Input: part model. Units: mm. Frame: model coordinates. A direction names the side the tool comes from. Give positions to 0.01 mm unless a question says otherwise; leave off trailing zeros. Loops run counter-clockwise (first coordinate to the right, second up) from the corner with the lowest first, then second, coordinate; pieces in that order, holes last. Notation, with made-up numbers: (68.25, -23.5) -> (101.25, -23.5) arc R21 cw to (101.25, 11.5) -> close; hole circle Ø8 at (43, -26.5). An arc over 180 degrees is marked (long way). Answer as a JSON object with one key per item and string values.
Autodesk Inventor part; units mm, degrees
ref_plane "Work Plane1" through (30.1625, 0, 0) normal (0, 0, -1) x (1, 0, 0)
ref_plane "YZ Plane" through (0, 0, 0) normal (1, 0, 0) x (0, 1, 0)
ref_plane "XZ Plane" through (0, 0, 0) normal (0, 1, 0) x (-1, 0, 0)
sketch "Sketch1" plane through (0, 0, 0) normal (0, 0, 1) x (1, 0, 0)
  line L0 (-7.1374, 0) -> (63.5, 0)
  line L1 (63.5, 0) -> (63.5, 6.35)
  line L2 (63.5, 6.35) -> (9.525, 6.35)
  line L3 (9.525, 6.35) -> (8.5483, 6.35)
  line L4 (8.5483, 6.35) -> (0, 6.35)
  line L5 (0, 6.35) -> (0, 12.5349)
  line L6 (-21.2649, 0) -> (77.6275, 0)
  line L7 (0, -2.507) -> (0, 15.0419)
  line L8 (-7.1374, 0) -> (-7.1374, 12.5349)
  line L9 (0, 12.5349) -> (-7.1374, 12.5349)
  line L10 (9.525, 6.35) -> (0, 6.35) construction
  dimension "d0" = 63.5
  dimension "d1" = 53.975
  dimension "d2" = 0.9767
  dimension "d3" = 7.1374
  dimension "d4" = 12.7
  dimension "d5" = 12.7
  dimension "d9" = 25.0698
  dimension "d10" = 0
revolve "Body" add sketch "Sketch1" angle 360 about axis through (-7.1374, 0, 0) along (1, 0, 0)
sketch "Sketch2" plane through (-7.1374, 0, 0) normal (-1, 0, 0) x (0, 0, 1)
  circle A0 centre (0, 0) radius 12.5349
  line L0 (0, 0) -> (0, 12.5349)
  line L1 (-12.5349, 1.3462) -> (12.5349, 1.3462)
  line L2 (12.5349, 1.3462) -> (12.5349, -1.3462)
  line L3 (12.5349, -1.3462) -> (-12.5349, -1.3462)
  line L4 (-12.5349, -1.3462) -> (-12.5349, 1.3462)
  line L5 (-12.5349, 0) -> (12.5349, 0) construction
  line L6 (0, 1.3462) -> (0, -1.3462) construction
  dimension "d11" = 2.6924
  dimension "d12" = 25.0698
fillet "Fillet1" radius 4.445 1 edges at (-7.1374, -12.5349, 0)
extrude "Slot" cut sketch "Sketch2" against normal blind 4.0894 contours A0 L3 L1 | L2 L3 A0 | A0 L1 L2 | L3 L4 A0 | A0 L4 L1
thread "Thread"
chamfer "Chamfer1" distance 0.9766 distance2 0.9767 1 edges at (63.5, -6.35, 0) measured on face at (63.5, 0.6891, 1.4726)
ref_plane "Work Plane1" through (30.1625, 0, 0) normal (0, 0, -1) x (1, 0, 0)
equation "\"d11\" = SBR"
equation "\"d12\" = KOD"
equation "\"d14\" = RR"
equation "\"d19\" = STI"
equation "\"d15\" = GEL"
equation "\"d17\" = -0.5 * SPD + 0.5 * GD"
equation "\"d0\" = NLG"
equation "\"d1\" = GEL"
equation "\"d3\" = KOH"
equation "\"d4\" = GD"
equation "\"d5\" = BDM"
equation "\"d9\" = KOD"
equation "\"GD\" = NND"
equation "\"NLG\" = 63.5"
equation "\"GEL\" = 53.975"
equation "\"KOD\" = 25.0698"
equation "\"KOH\" = 7.1374"
equation "\"GAL\" = 0.97663"
equation "\"SPD\" = GD1"
equation "\"BDM\" = NND"
equation "\"GUL\" = 0.97663"
equation "\"RR\" = 4.445"
equation "\"SBR\" = 2.6924"
equation "\"STI\" = 4.0894"
equation "\"KEWI\" = 0"
equation "\"THREADDIA\" = 12.7"
equation "\"TOA\" = 30deg"
equation "\"NND\" = 12.7"
equation "\"GD1\" = 10.74674"
properties part number "ANSI B18.6.3 - 1/2 - 13 x 2 1/2 SP HMS" material "Steel, Mild"
Q1. Access query for faces 4 (the flat face through (-3.048, 0, 0)), 5 (the flat face through (0, -6, 3)), 6 (the flat face through (-7.137, 4, 0)). Directions: +Z, -Z, +X, -X, +Y, -Y. A direction counts if a zero-diameter tool reaches every point of the face in a straight line with its end or side. Return the directions, or none.
Evaluation:
{"face 4": "+Z, -Z, -X", "face 5": "+X", "face 6": "+Z, -Z, -X, +Y, -Y"}
Q2. Section B-B, the plane z = 0. Return the cut outline in (x, y) (3 decimals).
Evaluation:
{"outline": "(-7.137, -8.09) arc R4.445 ccw to (-2.692, -12.535) -> (0, -12.535) -> (0, -6.35) -> (62.523, -6.35) -> (63.5, -5.373) -> (63.5, 5.373) -> (62.523, 6.35) -> (0, 6.35) -> (0, 12.535) -> (-2.692, 12.535) arc R4.445 ccw to (-7.137, 8.09) -> (-7.137, 1.346) -> (-3.048, 1.346) -> (-3.048, -1.346) -> (-7.137, -1.346) -> close"}
Q3. Draft query along Y for faces 1 (the flat face through (-5, 1.346, 0)), 2 (the flat face through (-7.137, -4, 0)), 3 (the cylindrical face through (30.82, -1.38, 6.2)). Return one class per face: +Y half, -Y half, draft (parallel to the pull), parting line (faces both ways), or undercut.
Evaluation:
{"face 1": "undercut", "face 2": "draft", "face 3": "parting line"}
Q4. Section C-C, the plane x = 24. Return the cut outline in (y, z).
Evaluation:
{"outline": "circle Ø12.7 at (0, 0)"}
Q5. Pin query (flat end, axial travel): pin 1 (8 mm diameter, centred on x = 36.5, y = -7, fed in from -Z); pin 2 (12 mm diameter, centred on y = -6.5, z = -6, fed in from -X); pin 3 (0.8 mm diameter, centred on y = 0, z = -6, fed in from -X); pin 4 (2 mm diameter, centred on x = 38, z = -0.5, fed in from -Y). Return the tip coordinate at first contact, or that it passes through.
Evaluation:
{"pin 1": "stops at z = -5.6", "pin 2": "stops at x = -7.14", "pin 3": "stops at x = -3.05", "pin 4": "stops at y = -6.35"}
Q6. Ray query, line 1 along X through (y, z) = (0, 9.75); line 2 along X through (y, z) = (-7.25, 2); line 3 along Z through (x, y) = (-1, -7.75). Return the intervals inside material, ascending.
Evaluation:
{"line 1": "x = -3.05 to 0", "line 2": "x = -7.14 to 0", "line 3": "z = -9.85 to 9.85"}
Q7. Section A-A, the plane y = 0. Return the cut outline in (x, z) (3 decimals), then the cut area to 3 significant figures.
Evaluation:
{"outline": "(-3.048, -12.521) arc R4.445 ccw to (-2.692, -12.535) -> (0, -12.535) -> (0, -6.35) -> (62.523, -6.35) -> (63.5, -5.373) -> (63.5, 5.373) -> (62.523, 6.35) -> (0, 6.35) -> (0, 12.535) -> (-2.692, 12.535) arc R4.445 ccw to (-3.048, 12.521) -> close", "area": "882 mm2"}
